Can you work these out from the model? Positions are in its coordinate system, mm. Face numbers are marked on the shaded views. A direction names the side the tool comes from. Give positions to 0.01 mm unless a question says otherwise; leave off trailing zeros. Loops run counter-clockwise (first coordinate to the right, second up) from the corner with the lowest first, then second, coordinate; pieces in that order, holes last. Notation, with made-up numbers: (69, 60.5) - (93, 60.5) arc R32 cw to (93, 93.5) - close; hole circle Ø10 at (28, 28). An arc over 180 degrees is marked (long way). Answer as a JSON object with one key per item and string values.
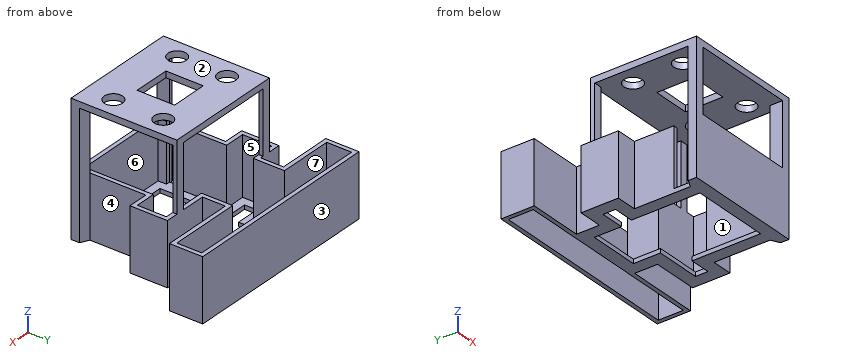
```python
from build123d import *

# Parameters (mm, degrees)
EXTRUDE_1_DEPTH      = 15
CUT_EXTRUDE_1_DEPTH  = 14
SKETCH_7_W           = 47
SKETCH_7_H           = 6
CUT_EXTRUDE_2_DEPTH  = 1
SKETCH_8_W           = 14
SKETCH_8_H           = 4
CUT_EXTRUDE_3_DEPTH  = 1
CUT_EXTRUDE_6_DEPTH  = 1
EXTRUDE_START        = -30
EXTRUDE_10_OUTLINE_W = 2
EXTRUDE_10_OUTLINE_H = 1
EXTRUDE_10_DEPTH     = 30
SKETCH_29_W          = 29
SKETCH_29_H          = 25.5
EXTRUDE_12_DEPTH     = 1.5
SKETCH_30_R          = 2.2
SKETCH_30_W          = 9
SKETCH_30_H          = 9
CUT_EXTRUDE_8_DEPTH  = 1.5


# Read off the part's stored shape, not the designer's step: 凸台-拉伸10
with BuildPart() as part:
    # 草图3 → 凸台-拉伸1 (new body)
    with BuildSketch(Plane.XY):
        Polygon((-25, 21.5), (24, 21.5), (24, 13.5), (6.5, 13.5), (6.5, 8), (17.5, 8), (17.5, -1), (12.5, -1), (12.5, -17.5), (-12.5, -17.5), (-12.5, -1), (-17.5, -1), (-17.5, 8), (-11.75, 8), (-11.75, 13.5), (-25, 13.5), align=None)
    extrude(amount=EXTRUDE_1_DEPTH)

    # 草图4 → 切除-拉伸1 (cut)
    with BuildSketch(Plane.XY.offset(15)):
        Polygon((23, 20.5), (-24, 20.5), (-24, 14.5), (-10.75, 14.5), (-10.75, 7), (-16.5, 7), (-16.5, 0), (-11.5, 0), (-11.5, -16.5), (11.5, -16.5), (11.5, 0), (16.5, 0), (16.5, 7), (5.5, 7), (5.5, 14.5), (23, 14.5), align=None)
    extrude(amount=-CUT_EXTRUDE_1_DEPTH, mode=Mode.SUBTRACT)

    # 草图7 → 切除-拉伸2 (cut)
    with BuildSketch(Plane.XY.offset(1)):
        with Locations((-0.5, 17.5)):
            Rectangle(SKETCH_7_W, SKETCH_7_H)
    extrude(amount=-CUT_EXTRUDE_2_DEPTH, mode=Mode.SUBTRACT)

    # 草图8 → 切除-拉伸3 (cut)
    with BuildSketch(Plane.ZY.offset(12.5)):
        with Locations((8, -12.5)):
            Rectangle(SKETCH_8_W, SKETCH_8_H)
    extrude(amount=-CUT_EXTRUDE_3_DEPTH, mode=Mode.SUBTRACT)

    # 草图9 → 切除-拉伸6 (cut)
    with BuildSketch(Plane(origin=(0, 0, 0), x_dir=(-1, 0, 0), z_dir=(0, 0, -1))):
        Polygon((-3.5, 11.5), (-3.5, 5), (-14.5, 5), (-14.5, 2), (-9.5, 2), (-9.5, -14.5), (9.5, -14.5), (9.5, 2), (14.5, 2), (14.5, 5), (8.75, 5), (8.75, 11.5), align=None)
    extrude(amount=-CUT_EXTRUDE_6_DEPTH, mode=Mode.SUBTRACT)

    # 凸台-拉伸10 outline → 凸台-拉伸10 (add)
    with BuildSketch(Plane(origin=(0, 0, 0), x_dir=(-1, 0, 0), z_dir=(0, 0, -1)).offset(EXTRUDE_START)):
        Polygon((-14.5, -17.5), (-12.5, -17.5), (-12.5, -14.5), (-14.5, -15.5), align=None)
        Polygon((12.5, -17.5), (14.5, -17.5), (14.5, -15.5), (12.5, -14.5), align=None)
        with Locations((-13.5, 7.5)):
            Rectangle(EXTRUDE_10_OUTLINE_W, EXTRUDE_10_OUTLINE_H)
        with Locations((13.5, 7.5)):
            Rectangle(EXTRUDE_10_OUTLINE_W, EXTRUDE_10_OUTLINE_H)
    extrude(amount=EXTRUDE_10_DEPTH)

    # 草图29 → 凸台-拉伸12 (add)
    with BuildSketch(Plane.XY.offset(30)):
        with Locations((0, -4.75)):
            Rectangle(SKETCH_29_W, SKETCH_29_H)
    extrude(amount=EXTRUDE_12_DEPTH)

    # 草图30 → 切除-拉伸8 (cut)
    with BuildSketch(Plane.XY.offset(31.5)):
        with Locations((-10, 1.25)):
            Circle(SKETCH_30_R)
        with Locations((-10, -10.75)):
            Circle(SKETCH_30_R)
        with Locations((10, 1.25)):
            Circle(SKETCH_30_R)
        with Locations((10, -10.75)):
            Circle(SKETCH_30_R)
        with Locations((0, -4.75)):
            Rectangle(SKETCH_30_W, SKETCH_30_H)
    extrude(amount=-CUT_EXTRUDE_8_DEPTH, mode=Mode.SUBTRACT)


solid = part.part
```
1) Imagine slicing it at C-C on y = 1.25. Write out the boundary of the cut face in (x, z).
Check sheet entries:
{"outline": "(-17.5, 0) - (-9.5, 0) - (-9.5, 1) - (-16.5, 1) - (-16.5, 15) - (-17.5, 15) - close; (-14.5, 30) - (-12.2, 30) - (-12.2, 31.5) - (-14.5, 31.5) - close; (-7.8, 30) - (7.8, 30) - (7.8, 31.5) - (-7.8, 31.5) - close; (9.5, 0) - (17.5, 0) - (17.5, 15) - (16.5, 15) - (16.5, 1) - (9.5, 1) - close; (12.2, 30) - (14.5, 30) - (14.5, 31.5) - (12.2, 31.5) - close"}
2) Which directions (+Z, -Z, +X, -X, +Y, -Y) give clear straight access to the entire face, cutting with the end or side of a thin tool? Please do the marked faces 4, 5, 6 and 7.
Check sheet entries:
{"face 4": "-Z, +X", "face 5": "+Z", "face 6": "none", "face 7": "+Z, -Z"}
3) Imagine slicing it at A-A on x = 1. Write out the boundary of the cut face in (y, z), and give its area (4 significant figures).
Check sheet entries:
{"outline": "(-17.5, 0) - (-14.5, 0) - (-14.5, 1) - (-16.5, 1) - (-16.5, 15) - (-17.5, 15) - close; (-17.5, 30) - (-9.25, 30) - (-9.25, 31.5) - (-17.5, 31.5) - close; (-0.25, 30) - (8, 30) - (8, 31.5) - (-0.25, 31.5) - close; (11.5, 0) - (14.5, 0) - (14.5, 1) - (11.5, 1) - close; (20.5, 0) - (21.5, 0) - (21.5, 15) - (20.5, 15) - close", "area": "59.75 mm2"}
4) I'm going to push flat-ended pins straight in: P1, Ø1.6, axis at x = -0.5, z = 31, coming from the +Y side; P2, Ø3.5, axis at y = 3.5, z = 9, coming from the +X side; P3, Ø1.6, axis at y = -2.5, z = 31, coming from the -X side. Where does each tip first touch, or does it pass through?
Check sheet entries:
{"P1": "y = 8", "P2": "x = 17.5", "P3": "x = -14.5"}
5) If we mould it in two halves opening along Z, with no side actions, what happens to the marked faces 1, 2 and 3? For each: released by +Z, released by -Z, zero draft, split by the parting line, or undercut.
Check sheet entries:
{"face 1": "undercut", "face 2": "released by +Z", "face 3": "zero draft"}
6) Imagine slicing it at B-B on z = 17. Write out the boundary of the cut face in (x, y).
Check sheet entries:
{"outline": "(-14.5, -17.5) - (-12.5, -17.5) - (-12.5, -14.5) - (-14.5, -15.5) - close; (-14.5, 7) - (-12.5, 7) - (-12.5, 8) - (-14.5, 8) - close; (12.5, -17.5) - (14.5, -17.5) - (14.5, -15.5) - (12.5, -14.5) - close; (12.5, 7) - (14.5, 7) - (14.5, 8) - (12.5, 8) - close"}
7) I need wall thicknesses on L1, parallel to X at y = 1, z = 31; L2, parallel to Y at x = 10, z = 30.4; L3, parallel to Y at x = 16, z = 4.5. Which ranges of each line are inside material? Lowest first, please.
Check sheet entries:
{"L1": "-14.5 to -12.19, -7.81 to 7.81, 12.19 to 14.5", "L2": "-17.5 to -12.95, -8.55 to -0.95, 3.45 to 8", "L3": "-1 to 0, 7 to 8, 13.5 to 14.5, 20.5 to 21.5"}
